Design review of the part built by this model. Coordinates are the model's own, in mm. Face numbers are marked on the shaded views. Give positions to 0.01 mm unless a question says otherwise; leave off trailing zeros. Order: outer loops, then holes, each group sorted by start corner. A loop starts at its lowest first (then second) coordinate and runs counter-clockwise, first axis right, second up. Notation, with made-up numbers: (16.5, 7) -> (44.5, 7) arc R20 ccw to (44.5, 23) -> close; hole circle Ø2 at (84, 15). An arc over 180 degrees is marked (long way). Use a Markdown table: item, result. Add a question column.
```python
from build123d import *

# Parameters (mm, degrees)
SKETCH1_R                                          = 2.55
SKETCH1_R_2                                        = 12.5
BOSS_EXTRUDE1_DEPTH                                = 10
CHAMBRAGE_POUR_VIS_T_TE_RONDE_BOMB_E_M_D           = 3.4
CHAMBRAGE_POUR_VIS_T_TE_RONDE_BOMB_E_M_CBORE_D     = 7
CHAMBRAGE_POUR_VIS_T_TE_RONDE_BOMB_E_M_CBORE_DEPTH = 3.5
DIAM_TRE_DU_PER_AGE_4_5_4_5_1_D                    = 4.5


with BuildPart() as part:
    # Sketch1 → Boss-Extrude1 (new body)
    # profile 1 of 3: a face of its own
    with BuildSketch(Plane.XY):
        with BuildLine():
            Line((15.75, 49), (-15.75, 49))
            ThreePointArc((-15.75, 49), (-18.578427125, 47.828427125), (-19.75, 45))
            Line((-19.75, 45), (-19.75, -45))
            ThreePointArc((-19.75, -45), (-18.578427125, -47.828427125), (-15.75, -49))
            Line((-15.75, -49), (15.75, -49))
            ThreePointArc((15.75, -49), (18.578427125, -47.828427125), (19.75, -45))
            Line((19.75, -45), (19.75, 45))
            ThreePointArc((19.75, 45), (18.578427125, 47.828427125), (15.75, 49))
        make_face()
        with Locations((0, -4.8)):
            Circle(SKETCH1_R, mode=Mode.SUBTRACT)
        with Locations((0, -24.8)):
            Circle(SKETCH1_R, mode=Mode.SUBTRACT)
        with Locations((0, 27.75)):
            Circle(SKETCH1_R_2, mode=Mode.SUBTRACT)
        with BuildLine():
            ThreePointArc((-16.596015511, 13.346015511), (-16.596015511, 11.153984489), (-14.403984489, 11.153984489))
            Line((-14.403984489, 11.153984489), (-11.903984489, 13.653984489))
            ThreePointArc((-11.903984489, 13.653984489), (-11.903984489, 15.846015511), (-14.096015511, 15.846015511))
            Line((-14.096015511, 15.846015511), (-16.596015511, 13.346015511))
        make_face(mode=Mode.SUBTRACT)
        with BuildLine():
            ThreePointArc((16.596015511, 42.153984489), (16.596015511, 44.346015511), (14.403984489, 44.346015511))
            Line((14.403984489, 44.346015511), (11.903984489, 41.846015511))
            ThreePointArc((11.903984489, 41.846015511), (11.903984489, 39.653984489), (14.096015511, 39.653984489))
            Line((14.096015511, 39.653984489), (16.596015511, 42.153984489))
        make_face(mode=Mode.SUBTRACT)
        with BuildLine():
            Line((-14.096015511, 39.653984489), (-16.596015511, 42.153984489))
            ThreePointArc((-16.596015511, 42.153984489), (-16.596015511, 44.346015511), (-14.403984489, 44.346015511))
            Line((-14.403984489, 44.346015511), (-11.903984489, 41.846015511))
            ThreePointArc((-11.903984489, 41.846015511), (-11.903984489, 39.653984489), (-14.096015511, 39.653984489))
        make_face(mode=Mode.SUBTRACT)
        with BuildLine():
            Line((14.096015511, 15.846015511), (16.596015511, 13.346015511))
            ThreePointArc((16.596015511, 13.346015511), (16.596015511, 11.153984489), (14.403984489, 11.153984489))
            Line((14.403984489, 11.153984489), (11.903984489, 13.653984489))
            ThreePointArc((11.903984489, 13.653984489), (11.903984489, 15.846015511), (14.096015511, 15.846015511))
        make_face(mode=Mode.SUBTRACT)
    # profile 2 of 3: a face of its own
    with BuildSketch(Plane.XY):
        with Locations((0, -24.8)):
            Circle(SKETCH1_R)
    # profile 3 of 3: a face of its own
    with BuildSketch(Plane.XY):
        with Locations((0, -4.8)):
            Circle(SKETCH1_R)
    extrude(amount=BOSS_EXTRUDE1_DEPTH)

    # Chambrage pour vis à tête ronde bombée M31 (through all)
    with Locations(Plane(origin=(0, 0, 0), x_dir=(1, 0, 0), z_dir=(0, 0, -1))):
        with Locations((0, 4.8), (0, 24.8)):
            CounterBoreHole(CHAMBRAGE_POUR_VIS_T_TE_RONDE_BOMB_E_M_D / 2, CHAMBRAGE_POUR_VIS_T_TE_RONDE_BOMB_E_M_CBORE_D / 2, CHAMBRAGE_POUR_VIS_T_TE_RONDE_BOMB_E_M_CBORE_DEPTH)

    # Diamètre du perçage Ø4.5 (4.5)1 (through all)
    with Locations(Plane(origin=(0, 0, 0), x_dir=(-1, 0, 0), z_dir=(0, 0, -1))):
        with Locations((-16.25, -35), (6.75, -45)):
            Hole(DIAM_TRE_DU_PER_AGE_4_5_4_5_1_D / 2)


solid = part.part
```
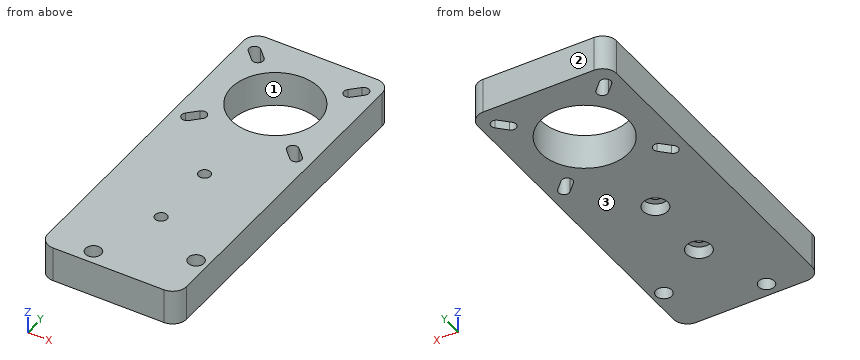
1) Insertion check: pin 1 (2 mm diameter, centred on x = 0, y = -24.8, fed in from +Z); pin 2 (6.5 mm diameter, centred on x = 0, y = -4.8, fed in from -Z). Each pin has a flat end and moves straight along its axis. Give the tip position at first contact, or say it passes through.
2) Add section B-B (y = -35). Give the boundary of the cut face in (x, z).
3) Add section C-C (z = 7.5). Give the number of separate pieces and of enclosed holes in the cut face, then the cut area to 3 significant figures.
4) For L1, parallel to Y at x = 0, z = 1.2; L2, parallel to Y at x = 0, z = 7; L3, parallel to Y at x = -16.5, z = 0.75, list the stretches that pass through material, from the lowest coordinate up. Write a range as [from, to].
5) Add section D-D (x = -6.75). Give the boundary of the cut face in (y, z), then the cut area to 3 significant figures.
6) The part is to be moulded in two halves that separate along Y. For the marked faces 1, 2 and 3, say which applies: +Y half, -Y half, draft (parallel to the pull), parting line (faces both ways), or undercut.
7) Add section A-A (x = 0). Give the boundary of the cut face in (y, z).
Worked answers:
| question | item | result |
|---|---|---|
| 1 | pin 1 | through |
| 1 | pin 2 | z = 3.5 |
| 2 | outline | (-19.75, 0) -> (14, 0) -> (14, 10) -> (-19.75, 10) -> close; (18.5, 0) -> (19.75, 0) -> (19.75, 10) -> (18.5, 10) -> close |
| 3 | separate pieces | 1 |
| 3 | enclosed holes | 9 |
| 3 | area | 3,240 mm^2 |
| 4 | L1 | [-49, -28.3], [-21.3, -8.3], [-1.3, 15.25], [40.25, 49] |
| 4 | L2 | [-49, -26.5], [-23.1, -6.5], [-3.1, 15.25], [40.25, 49] |
| 4 | L3 | [-48.93, 11.07], [13.44, 42.06], [44.43, 48.93] |
| 5 | outline | (-49, 0) -> (-47.25, 0) -> (-47.25, 10) -> (-49, 10) -> close; (-42.75, 0) -> (17.23, 0) -> (17.23, 10) -> (-42.75, 10) -> close; (38.27, 0) -> (49, 0) -> (49, 10) -> (38.27, 10) -> close |
| 5 | area | 725 mm^2 |
| 6 | face 1 | undercut |
| 6 | face 2 | +Y half |
| 6 | face 3 | draft |
| 7 | outline | (-49, 0) -> (-28.3, 0) -> (-28.3, 3.5) -> (-26.5, 3.5) -> (-26.5, 10) -> (-49, 10) -> close; (-23.1, 3.5) -> (-21.3, 3.5) -> (-21.3, 0) -> (-8.3, 0) -> (-8.3, 3.5) -> (-6.5, 3.5) -> (-6.5, 10) -> (-23.1, 10) -> close; (-3.1, 3.5) -> (-1.3, 3.5) -> (-1.3, 0) -> (15.25, 0) -> (15.25, 10) -> (-3.1, 10) -> close; (40.25, 0) -> (49, 0) -> (49, 10) -> (40.25, 10) -> close |
